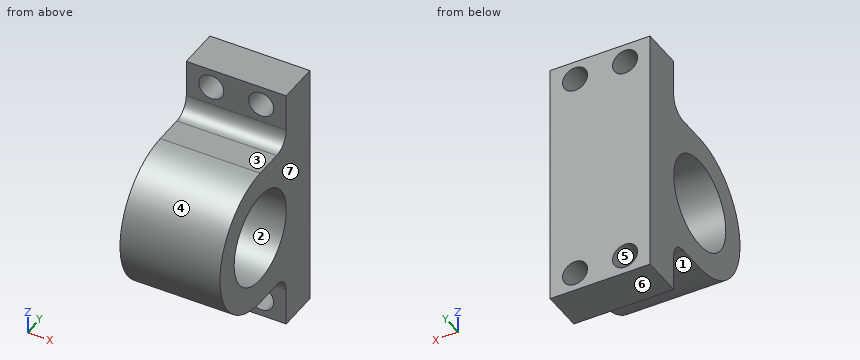
from build123d import *

# Parameters (mm, degrees)
SKETCH_2_R          = 5.5
EXTRUDE_1_DEPTH     = 12
SKETCH_5_R          = 1.5
CUT_EXTRUDE_1_DEPTH = 5


with BuildPart() as part:
    # 草图2 → 凸台-拉伸1 (new body)
    with BuildSketch(Plane(origin=(0, 0, 0), x_dir=(0, 0, -1), z_dir=(1, 0, 0))):
        with BuildLine():
            Line((-15, 5.5), (-15, 10.5))
            Line((-15, 10.5), (15, 10.5))
            Line((15, 10.5), (15, 5.5))
            Line((15, 5.5), (10.5, 5.5))
            ThreePointArc((10.5, 5.5), (9.085786438, 4.914213562), (8.5, 3.5))
            Line((8.5, 3.5), (8.5, 0))
            ThreePointArc((8.5, 0), (0, -8.5), (-8.5, 0))
            Line((-8.5, 0), (-8.5, 3.5))
            ThreePointArc((-8.5, 3.5), (-9.085786438, 4.914213562), (-10.5, 5.5))
            Line((-10.5, 5.5), (-15, 5.5))
        make_face()
        Circle(SKETCH_2_R, mode=Mode.SUBTRACT)
    extrude(amount=EXTRUDE_1_DEPTH)

    # 草图5 → 切除-拉伸1 (cut)
    with BuildSketch(Plane.XZ.offset(-5.5)):
        with Locations(Location((3, 12.75, 0), (0, 0, 270))):
            Circle(SKETCH_5_R)
        with Locations(Location((9, 12.75, 0), (0, 0, 270))):
            Circle(SKETCH_5_R)
        with Locations(Location((9, -12.75, 0), (0, 0, 270))):
            Circle(SKETCH_5_R)
        with Locations(Location((3, -12.75, 0), (0, 0, 270))):
            Circle(SKETCH_5_R)
    extrude(amount=-CUT_EXTRUDE_1_DEPTH, mode=Mode.SUBTRACT)


solid = part.part
Geometry: final body of the model. Coordinates: model frame, mm. Face numbers are marked on the shaded views. A direction names the side the tool comes from. Round coordinates to 2 decimals unless told otherwise and drop trailing zeros. Loops run counter-clockwise (first coordinate to the right, second up) from the corner with the lowest first, then second, coordinate; pieces in that order, holes last.
Q1. Section A-A on x = 9. Return loops of the section in (y, z).
Q2. Pin query (flat end, axial travel): P1, Ø1.3, axis at x = 5.5, z = 12.5, coming from the -Y side; P2, Ø4, axis at x = 6.5, y = 0.5, coming from the +Z side; P3, Ø3, axis at x = 4.5, y = 1.5, coming from the -Z side. Return the tip coordinate at first contact, or that it passes through.
Q3. Section B-B on z = 0. Return loops of the section in (x, y), plus the area to 3 significant figures.
Q4. Material intervals for L1, parallel to X at y = 7.75, z = 12.75; L2, parallel to Y at x = 4.75, z = 0; L3, parallel to Z at x = 5, y = -0.25, sorted ascending.
Q5. Section D-D on x = 7. Return loops of the section in (y, z), plus the area to 3 significant figures.
Q6. Access query for the marked faces 1, 2 and 3. Directions: +Z, -Z, +X, -X, +Y, -Y. A direction counts if a zero-diameter tool reaches every point of the face in a straight line with its end or side. Return the directions, or none.
Q7. Section C-C on y = -0.5. Return loops of the section in (x, z).
Q8. Pull-direction query (Z, two-part tool) for the marked faces 4, 5, 6 and 7; classes: released by +Z, released by -Z, zero draft, split by the parting line, or undercut.
Evaluation:
1. outline: (0, -8.5) - (3.5, -8.5) arc R2 cw to (5.5, -10.5) - (5.5, -11.25) - (10.5, -11.25) - (10.5, 11.25) - (5.5, 11.25) - (5.5, 10.5) arc R2 cw to (3.5, 8.5) - (0, 8.5) arc R8.5 ccw to start; (5.5, -15) - (10.5, -15) - (10.5, -14.25) - (5.5, -14.25) - close; (5.5, 14.25) - (10.5, 14.25) - (10.5, 15) - (5.5, 15) - close; hole circle Ø11 at (0, 0)
2. P1: stops at y = 5.5
2. P2: stops at z = 8.5
2. P3: stops at z = -8.5
3. outline: (0, -8.5) - (12, -8.5) - (12, -5.5) - (0, -5.5) - close; (0, 5.5) - (12, 5.5) - (12, 10.5) - (0, 10.5) - close
3. area: 96.0 mm2
4. L1: x = 0 to 1.5, 4.5 to 7.5, 10.5 to 12
4. L2: y = -8.5 to -5.5, 5.5 to 10.5
4. L3: z = -8.5 to -5.49, 5.49 to 8.5
5. outline: (0, -8.5) - (3.5, -8.5) arc R2 cw to (5.5, -10.5) - (5.5, -15) - (10.5, -15) - (10.5, 15) - (5.5, 15) - (5.5, 10.5) arc R2 cw to (3.5, 8.5) - (0, 8.5) arc R8.5 ccw to start; hole circle Ø11 at (0, 0)
5. area: 264 mm2
6. face 1: -Z, +X, -X, -Y
6. face 2: +X, -X
6. face 3: +Z, +X, -X, -Y
7. outline: (0, -8.49) - (12, -8.49) - (12, -5.48) - (0, -5.48) - close; (0, 5.48) - (12, 5.48) - (12, 8.49) - (0, 8.49) - close
8. face 4: split by the parting line
8. face 5: undercut
8. face 6: released by -Z
8. face 7: zero draft
